Autodesk Inventor part; units mm, degrees
ref_plane "YZ Plane" through (0, 0, 0) normal (1, 0, 0) x (0, 1, 0)
ref_plane "XZ Plane" through (0, 0, 0) normal (0, 1, 0) x (-1, 0, 0)
ref_plane "XY Plane" through (0, 0, 0) normal (0, 0, 1) x (1, 0, 0)
sketch "Sketch1" plane through (0, 0, 0) normal (0, 0, 1) x (1, 0, 0)
  line L0 (0, 80) -> (0, 0)
  line L1 (0, 0) -> (70, 0)
  line L2 (70, 0) -> (70, 80)
  line L3 (6, 80) -> (6, 6)
  line L4 (6, 6) -> (64, 6)
  line L5 (64, 6) -> (64, 80)
  line L6 (0, 80) -> (6, 80)
  line L7 (64, 80) -> (70, 80)
  dimension "d0" = 70
  dimension "d1" = 80
  dimension "d2" = 80
  dimension "d3" = 6
extrude "Extrusion1" add sketch "Sketch1" along normal blind 50
sketch "Sketch2" plane through (0, 0, 0) normal (0, -1, 0) x (1, 0, 0)
  line L0 (6, 0) -> (0, 0)
  line L1 (0, 50) -> (70, 50)
  line L2 (0, 0) -> (70, 0)
  line L3 (70, 0) -> (70, 50)
  line L4 (70, 50) -> (0, 50)
  line L5 (0, 50) -> (0, 0)
  line L6 (6, 6) -> (64, 6)
  line L7 (64, 6) -> (64, 44)
  line L8 (64, 44) -> (6, 44)
  line L9 (6, 44) -> (6, 6)
  dimension "d7" = 6
extrude "Extrusion2" add sketch "Sketch2" along normal blind 40
sketch "Sketch3" plane through (0, 0, 50) normal (0, 0, 1) x (1, 0, 0)
  line L0 (70, 80) -> (70, -40)
  line L1 (70, -40) -> (0, -40)
  line L2 (0, -40) -> (0, -47)
  line L3 (0, -47) -> (70, -47)
  line L4 (70, -47) -> (70, -40)
  point P0 (0, 0)
  dimension "d15" = 70
  dimension "d16" = 7
extrude "Extrusion4" add sketch "Sketch3" against normal blind 50
properties part number "armj4"
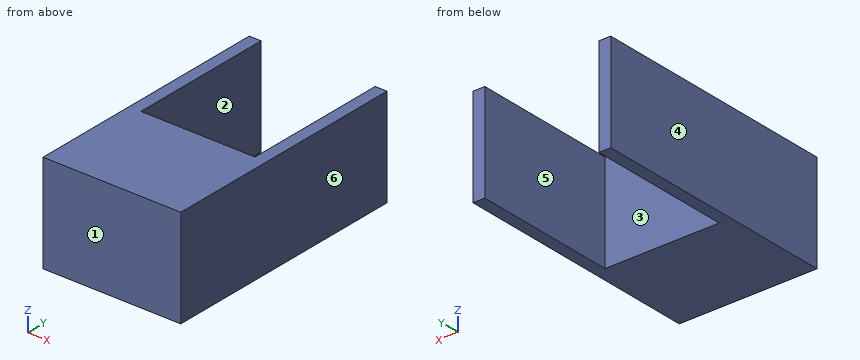
Verification items for the finished model (mm, model axes). Face numbers are marked on the shaded views. A direction names the side the tool comes from. Coordinates: 2 decimals unless noted, no trailing zeros. Order: outer loops, then holes, each group sorted by start corner. A loop starts at its lowest first (then second) coordinate and runs counter-clockwise, first axis right, second up. Notation, with made-up numbers: (62.25, -27.75) -> (115.25, -27.75) arc R22 cw to (115.25, -16.75) -> close; hole circle Ø9 at (-11.5, 30). An arc over 180 degrees is marked (long way). Put each result on its own line as item: value. Start each with the question number.
1. Access from +Z, -Z, +X, -X, +Y, -Y to the whole of each face (thin tool, end or side, straight path). Record for the marked faces 5 and 6.
2. Material ranges on L1, parallel to Y at x = 27.5, z = 8; L2, parallel to X at y = 47, z = 24; L3, parallel to Z at x = 12, y = -21.5, recorded low to high. Write a range as [from, to].
3. Cross-section at C-C, the plane y = 15.5. Record the boundary of the cut face in (x, z).
4. Go/stop test with a flat-tipped pin: pin 1 Ø12 at (x, z) = (54, 29) entering from +Y. Record where the tip stops, or that it passes through.
5. Mould release check, pull along X, two halves, no side actions. Record for the marked faces 1, 2, 3 and 4: released by +X, released by -X, zero draft, split by the parting line, or undercut.
6. Cross-section at A-A, the plane z = 9. Record the boundary of the cut face in (x, y), then the cut area to 3 significant figures.
7. Cross-section at D-D, the plane x = 33.5. Record the boundary of the cut face in (y, z).
8. Cross-section at B-B, the plane y = -11. Record the boundary of the cut face in (x, z).
Computed:
1. face 5: +Z, -Z, +Y
1. face 6: +Z, -Z, +X, +Y, -Y
2. L1: [-47, -40], [0, 6]
2. L2: [0, 6], [64, 70]
2. L3: [0, 6], [44, 50]
3. outline: (0, 0) -> (6, 0) -> (6, 50) -> (0, 50) -> close; (64, 0) -> (70, 0) -> (70, 50) -> (64, 50) -> close
4. pin 1: y = 6
5. face 1: zero draft
5. face 2: undercut
5. face 3: undercut
5. face 4: released by -X
6. outline: (0, -47) -> (70, -47) -> (70, 80) -> (64, 80) -> (64, 6) -> (6, 6) -> (6, 80) -> (0, 80) -> close; hole (6, -40) -> (64, -40) -> (64, 0) -> (6, 0) -> close
6. area: 2,280 mm2
7. outline: (-47, 0) -> (6, 0) -> (6, 50) -> (-47, 50) -> close; hole (-40, 6) -> (0, 6) -> (0, 44) -> (-40, 44) -> close
8. outline: (0, 0) -> (70, 0) -> (70, 50) -> (0, 50) -> close; hole (6, 6) -> (64, 6) -> (64, 44) -> (6, 44) -> close
